Build history of the part. All positions in model axes, mm. Round coordinates to 2 decimals unless told otherwise and drop trailing zeros. Write each loop counter-clockwise with the first axis right and the second up, starting at its lowest first coordinate (ties: lowest second). Pieces come first, ordered by that corner, then holes. Notation, with made-up numbers: (24.25, -7) -> (41.25, -7) arc R13 ccw to (41.25, 10) -> close; hole circle Ø1 at (0.25, 45). An arc over 180 degrees is marked (long way). Answer in a Markdown table with one row per item.
```python
from build123d import *

# Parameters (mm, degrees)
SKETCH1_R           = 6.35
SKETCH1_R_2         = 2.4892
BOSS_EXTRUDE1_DEPTH = 3.175
FILLET1_R           = 6.35


with BuildPart() as part:
    # Sketch1 → Boss-Extrude1 (new body)
    with BuildSketch(Plane.XY):
        Polygon((0, 26.9875), (23.371860585, -13.49375), (-23.371860585, -13.49375), align=None)
        Circle(SKETCH1_R, mode=Mode.SUBTRACT)
        with Locations((0, 14.2875)):
            Circle(SKETCH1_R_2, mode=Mode.SUBTRACT)
        with Locations((12.373337957, -7.14375)):
            Circle(SKETCH1_R_2, mode=Mode.SUBTRACT)
        with Locations((-12.373337957, -7.14375)):
            Circle(SKETCH1_R_2, mode=Mode.SUBTRACT)
    extrude(amount=BOSS_EXTRUDE1_DEPTH)

    # Fillet1
    fillet1_edges = [part.edges().sort_by_distance(p)[0] for p in [
        (0, 26.9875, 1.5875),
        (23.371860585, -13.49375, 1.5875),
        (-23.371860585, -13.49375, 1.5875),
    ]]
    fillet(fillet1_edges, radius=FILLET1_R)


solid = part.part
```
Q1. Saw through at A-A on x = 0. State how many separate pieces and enclosed holes the cut face has, plus the area to 3 significant figures.
A:
| item | result |
|---|---|
| separate pieces | 3 |
| enclosed holes | 0 |
| area | 52.2 mm² |
Q2. Two-plate mould, pull along Y, no slides. Class faces 1 (the cylindrical face through (-17.919, -10.238, 1.61)), 2 (the cylindrical face through (-0.54, 11.857, 1.565)), 3 (the cylindrical face through (0.093, 20.637, 1.61)): released by +Y, released by -Y, zero draft, split by the parting line, or undercut.
A:
| item | result |
|---|---|
| face 1 | split by the parting line |
| face 2 | undercut |
| face 3 | released by +Y |
Q3. Wall check: line 1 (X direction, y = -7, z = 0.5); line 2 (X direction, y = -6.5, z = 0.55); line 3 (X direction, y = -4.5, z = 1.9). Give the ranges that are in metal, low to high. Write a range as [from, to].
A:
| item | result |
|---|---|
| line 1 | [-18.72, -14.86], [-9.89, 9.89], [14.86, 18.72] |
| line 2 | [-18.69, -14.78], [-9.97, 9.97], [14.78, 18.69] |
| line 3 | [-18.15, -4.48], [4.48, 18.15] |
Q4. Drop a flat-ended pin along its axis: P1, Ø1.5, axis at x = 13.5, z = 0.5, coming from the -Y side. Give the stop position or say it passes through.
A:
| item | result |
|---|---|
| P1 | y = -13.48 |
Q5. Saw through at B-B on y = -2.5. Write the cut outline in (x, z) (3 decimals).
A:
| item | result |
|---|---|
| outline | (-17.025, 0) -> (-5.837, 0) -> (-5.837, 3.175) -> (-17.025, 3.175) -> close; (5.837, 0) -> (17.025, 0) -> (17.025, 3.175) -> (5.837, 3.175) -> close |
Q6. Saw through at C-C on z = 2.6. Write the cut outline in (x, y), plus the area to 3 significant figures.
A:
| item | result |
|---|---|
| outline | (-17.87, -3.97) arc R6.35 ccw to (-12.37, -13.49) -> (12.37, -13.49) arc R6.35 ccw to (17.87, -3.97) -> (5.5, 17.46) arc R6.35 ccw to (-5.5, 17.46) -> close; hole circle Ø4.98 at (-12.37, -7.14); hole circle Ø12.7 at (0, 0); hole circle Ø4.98 at (0, 14.29); hole circle Ø4.98 at (12.37, -7.14) |
| area | 678 mm² |
Q7. Saw through at D-D on x = -13. Write the cut outline in (y, z) (3 decimals).
A:
| item | result |
|---|---|
| outline | (-13.463, 0) -> (-9.553, 0) -> (-9.553, 3.175) -> (-13.463, 3.175) -> close; (-4.735, 0) -> (4.471, 0) -> (4.471, 3.175) -> (-4.735, 3.175) -> close |
